Verification items for this drawing (mm, ordinates from the low corner). Round coordinates to 2 decimals unless told otherwise and drop trailing zeros. Order: outer loops, then holes, each group sorted by start corner. A loop starts at its lowest first (then second) coordinate and runs counter-clockwise, first axis right, second up. Notation, with made-up numbers: M 8.5,89 L 48.5,89 A28 cw 48.5,128 Z; hole C 23,21.5 d2. An arc over 180 degrees is marked long. Use CSV: the item, a comma, the result in double quotes. Start each with the question number.
Q1. Sectioned sample at B-B (y = 20.5). Enter the section's corners in (x, z).
Q2. Scan lines: line 1 (Y direction, x = 44.5, z = 22); line 2 (X direction, y = 10, z = 51); line 3 (Y direction, x = 70.5, z = 19) (1 decimal). Record each from-to range of solid material in increasing order.
Q3. Sectioned sample at A-A (x = 38.1). Enter the section's corners in (y, z) (1 decimal), and give its area (3 significant figures).
Q4. Gauge pin test, flat ends, axial feed: pin 1 Ø1 at (x, y) = (24.5, 47) entering from -Z; pin 2 Ø8 at (y, z) = (5.5, 67.5) entering from +X; pin 3 Ø8 at (x, y) = (20.5, 39) entering from +Z. Record the tip position at first contact, or that the pin passes through.
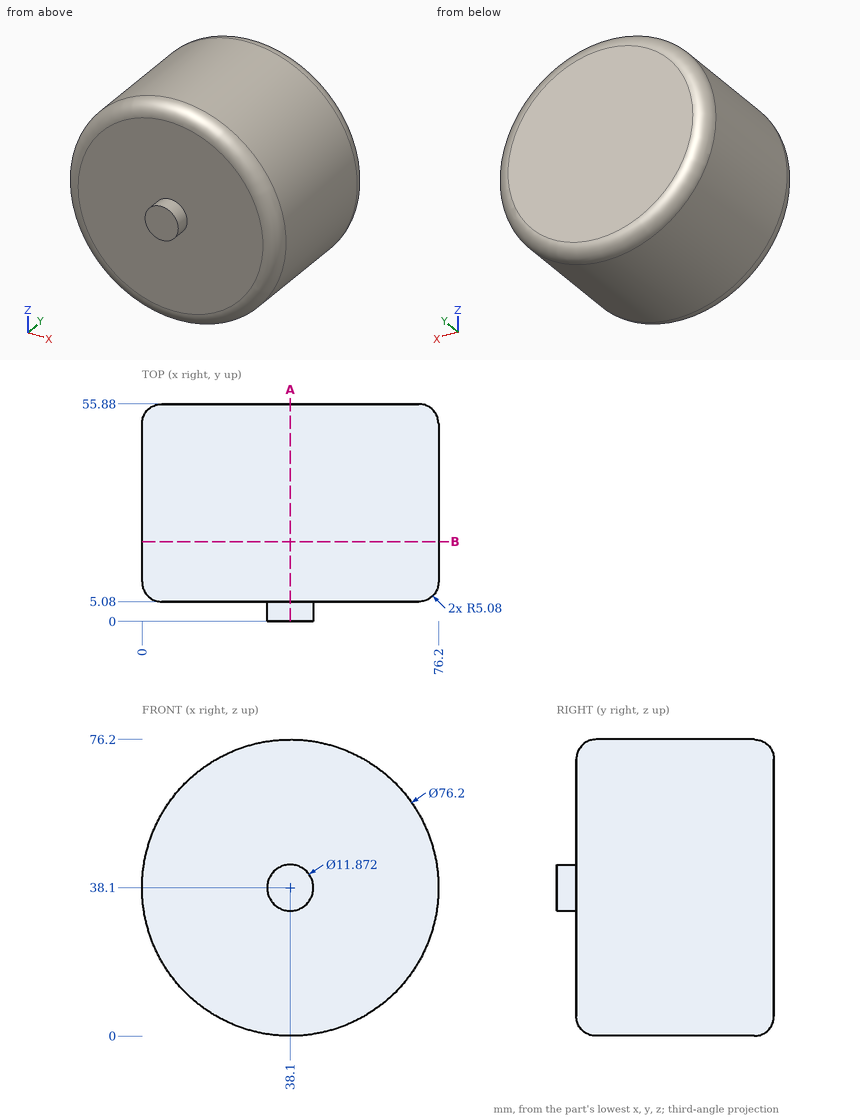
Verdict:
1,outline,"C 38.1,38.1 d76.2"
2,line 1,"y = 5.08 to 55.88"
2,line 2,"x = 2.25 to 73.95"
2,line 3,"y = 8 to 53"
3,outline,"M 0,32.2 L 5.1,32.2 L 5.1,5.1 A5.1 ccw 10.2,0 L 50.8,0 A5.1 ccw 55.9,5.1 L 55.9,71.1 A5.1 ccw 50.8,76.2 L 10.2,76.2 A5.1 ccw 5.1,71.1 L 5.1,44 L 0,44 Z"
3,area,"3,910 mm²"
4,pin 1,"stops at z = 2.32"
4,pin 2,"stops at x = 65.03"
4,pin 3,"stops at z = 73.69"
